Check sheet for the modelled part. Datum: model origin and axes. Units: mm. Face numbers are marked on the shaded views. Coordinates: 2 decimals unless noted, no trailing zeros. Write each loop counter-clockwise with the first axis right and the second up, starting at its lowest first coordinate (ties: lowest second). Pieces come first, ordered by that corner, then holes. Notation, with made-up numbers: (-36, 84) -> (12, 84) arc R7 cw to (12, 88) -> close; hole circle Ø11 at (30.25, 76). An arc over 180 degrees is marked (long way). One line per item, written item: value. Start each with the question number.
1) Sectioned sample at C-C on z = 3. Enter the section's corners in (x, y).
2) Draft check along X on the marked faces 1, 2 and 3. Enter one of: +X half, -X half, draft (parallel to the pull), parting line (faces both ways), or undercut.
3) Sectioned sample at B-B on y = 37. Enter the section's corners in (x, z), plus the area to 3 significant figures.
4) Sectioned sample at D-D on x = 37. Enter the section's corners in (y, z), plus the area to 3 significant figures.
5) Sectioned sample at A-A on x = 30. Enter the section's corners in (y, z).
6) Scan lines: line 1 along Y through (x, z) = (20, -1.6); line 2 along Y through (x, z) = (18.5, -0.5); line 3 along X through (y, z) = (-33.5, 1.75). Record each from-to range of solid material in increasing order. Write a range as [from, to].
7) Gauge pin test, flat ends, axial feed: P1, Ø15.5, axis at x = 35, y = -35, coming from the +Z side; P2, Ø9.5, axis at x = 20, y = 37, coming from the +Z side; P3, Ø20, axis at x = 24.5, y = 5, coming from the -Z side; P4, Ø1.5, axis at y = -20, z = -1.5, coming from the -X side. Record the tip position at first contact, or that the pin passes through.
```python
from build123d import *

# Parameters (mm, degrees)
SKETCH1_R           = 3.25
SKETCH1_R_2         = 6
BOSS_EXTRUDE1_DEPTH = 4
SKETCH3_R           = 36
CUT_EXTRUDE2_DEPTH  = 3
FILLET1_R           = 5
SKETCH4_R           = 6
CUT_EXTRUDE3_DEPTH  = 4


with BuildPart() as part:
    # Sketch1 → Boss-Extrude1 (new body, symmetric)
    with BuildSketch(Plane.XY):
        with BuildLine():
            Line((45, -45), (11, -45))
            Line((11, -45), (11, -32.435512945))
            ThreePointArc((11, -32.435512945), (34.25, 0), (11, 32.435512945))
            Line((11, 32.435512945), (11, 45))
            Line((11, 45), (45, 45))
            Line((45, 45), (45, -45))
        make_face()
        with Locations((20, 37)):
            Circle(SKETCH1_R, mode=Mode.SUBTRACT)
        with Locations((35, 35)):
            Circle(SKETCH1_R_2, mode=Mode.SUBTRACT)
        with Locations((37, 20)):
            Circle(SKETCH1_R, mode=Mode.SUBTRACT)
        with Locations((37, -20)):
            Circle(SKETCH1_R, mode=Mode.SUBTRACT)
        with Locations((35, -35)):
            Circle(SKETCH1_R_2, mode=Mode.SUBTRACT)
        with Locations((20, -37)):
            Circle(SKETCH1_R, mode=Mode.SUBTRACT)
    extrude(amount=BOSS_EXTRUDE1_DEPTH, both=True)

    # Sketch3 → Cut-Extrude2 (cut)
    with BuildSketch(Plane(origin=(0, 0, -4), x_dir=(-1, 0, 0), z_dir=(0, 0, -1))):
        Circle(SKETCH3_R)
    extrude(amount=-CUT_EXTRUDE2_DEPTH, mode=Mode.SUBTRACT)

    # Fillet1
    fillet1_edges = [part.edges().sort_by_distance(p)[0] for p in [
        (45, 45, 0),
        (45, -45, 0),
    ]]
    fillet(fillet1_edges, radius=FILLET1_R)

    # Sketch4 → Cut-Extrude3 (cut)
    with BuildSketch(Plane.XY.offset(4)):
        with Locations((20, 37)):
            Circle(SKETCH4_R)
        with Locations((37, 20)):
            Circle(SKETCH4_R)
        with Locations((20, -37)):
            Circle(SKETCH4_R)
        with Locations((37, -20)):
            Circle(SKETCH4_R)
    extrude(amount=-CUT_EXTRUDE3_DEPTH, mode=Mode.SUBTRACT)


solid = part.part
```
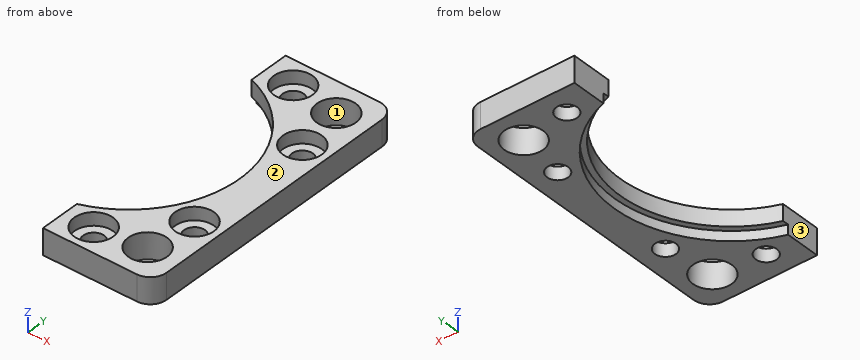
Answers:
1. outline: (11, -45) -> (40, -45) arc R5 ccw to (45, -40) -> (45, 40) arc R5 ccw to (40, 45) -> (11, 45) -> (11, 32.44) arc R34.25 cw to (11, -32.44) -> close; hole circle Ø12 at (20, -37); hole circle Ø12 at (20, 37); hole circle Ø12 at (35, -35); hole circle Ø12 at (35, 35); hole circle Ø12 at (37, -20); hole circle Ø12 at (37, 20)
2. face 1: undercut
2. face 2: draft
2. face 3: -X half
3. outline: (11, -4) -> (16.75, -4) -> (16.75, 0) -> (14, 0) -> (14, 4) -> (11, 4) -> close; (23.25, -4) -> (29.34, -4) -> (29.34, 4) -> (26, 4) -> (26, 0) -> (23.25, 0) -> close; (40.66, -4) -> (45, -4) -> (45, 4) -> (40.66, 4) -> close
3. area: 107 mm2
4. outline: (-45, -4) -> (-40.66, -4) -> (-40.66, 4) -> (-45, 4) -> close; (-29.34, -4) -> (-23.25, -4) -> (-23.25, 0) -> (-26, 0) -> (-26, 4) -> (-29.34, 4) -> close; (-16.75, -4) -> (16.75, -4) -> (16.75, 0) -> (14, 0) -> (14, 4) -> (-14, 4) -> (-14, 0) -> (-16.75, 0) -> close; (23.25, -4) -> (29.34, -4) -> (29.34, 4) -> (26, 4) -> (26, 0) -> (23.25, 0) -> close; (40.66, -4) -> (45, -4) -> (45, 4) -> (40.66, 4) -> close
4. area: 391 mm2
5. outline: (-45, -4) -> (-38.32, -4) -> (-38.32, 4) -> (-45, 4) -> close; (-31.68, -4) -> (-19.9, -4) -> (-19.9, -1) -> (-16.52, -1) -> (-16.52, 4) -> (-31.68, 4) -> close; (16.52, -1) -> (19.9, -1) -> (19.9, -4) -> (31.68, -4) -> (31.68, 4) -> (16.52, 4) -> close; (38.32, -4) -> (45, -4) -> (45, 4) -> (38.32, 4) -> close
6. line 1: y = [-45, -40.25], [-33.75, -29.93], [29.93, 33.75], [40.25, 45]
6. line 2: y = [-45, -39.88], [-34.12, -28.82], [28.82, 34.12], [39.88, 45]
6. line 3: x = [11, 15.13], [24.87, 29.19], [40.81, 45]
7. P1: stops at z = 4
7. P2: stops at z = 0
7. P3: stops at z = -1
7. P4: stops at x = 27.39
